Geometry check sheet. Reference: drawing and pictorial views, mm from the part's lowest x, y, z. Round coordinates to 2 decimals unless told otherwise and drop trailing zeros. Write each loop counter-clockwise with the first axis right and the second up, starting at its lowest first coordinate (ties: lowest second). Pieces come first, ordered by that corner, then holes.
Item 1: Section check A-A, the plane z = 39. Record the cut outline in (x, y) (3 decimals).
Item 2: Section check C-C, the plane z = 56. Record the cut outline in (x, y) (3 decimals).
Item 3: Depth check by flat-ended pin: pin 1 (1.5 mm diameter, centred on y = 1, z = 25, fed in from -X); pin 2 (1.9 mm diameter, centred on y = 2, z = 52, fed in from -X); pin 3 (3 mm diameter, centred on y = 2, z = 53, fed in from +X). Enter the tip coordinate at first touch or a pass-through.
Item 4: Section check B-B, the plane y = 4.5. Record the cut outline in (x, z) (3 decimals), plus the area to 3 significant figures.
Item 5: Section check D-D, the plane x = 49. Record the cut outline in (y, z).
Item 6: Material ranges on line 1 along X through (y, z) = (1.5, 30) (3 decimals); line 2 along X through (y, z) = (5.5, 62) (3 decimals); line 3 along Z through (x, y) = (55, 2.25), recorded low to high.
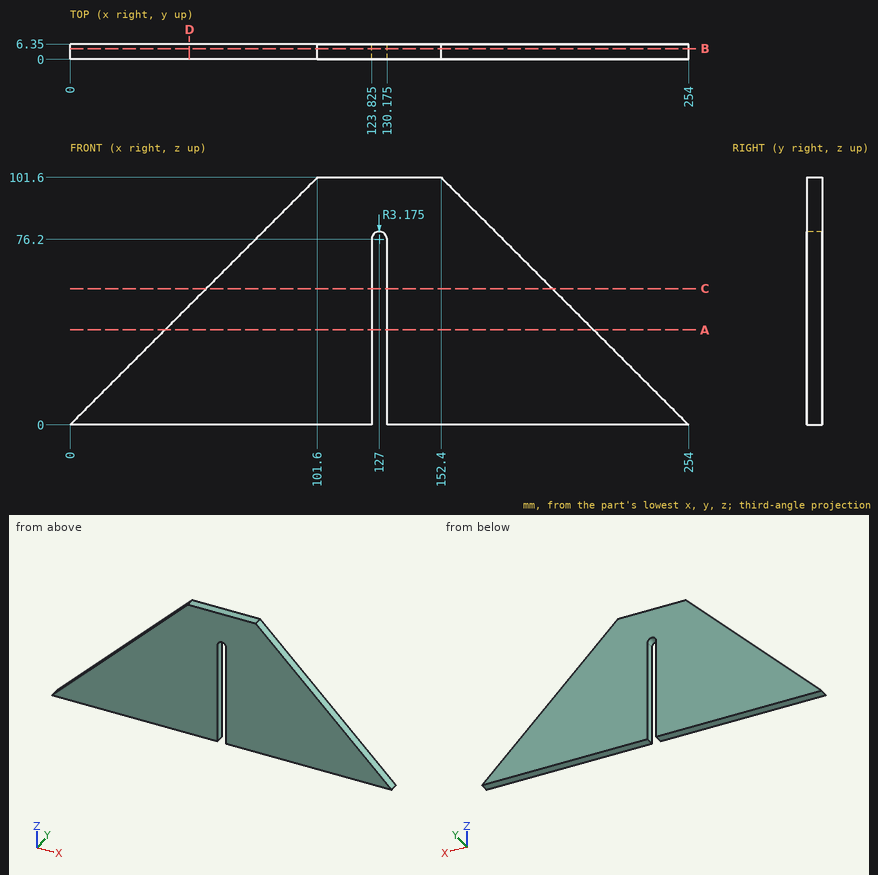
Values found:
1. outline: (39, 0) - (123.825, 0) - (123.825, 6.35) - (39, 6.35) - close; (130.175, 0) - (215, 0) - (215, 6.35) - (130.175, 6.35) - close
2. outline: (56, 0) - (123.825, 0) - (123.825, 6.35) - (56, 6.35) - close; (130.175, 0) - (198, 0) - (198, 6.35) - (130.175, 6.35) - close
3. pin 1: stops at x = 24.25
3. pin 2: stops at x = 51.05
3. pin 3: stops at x = 202.5
4. outline: (0, 0) - (123.825, 0) - (123.825, 76.2) arc R3.175 cw to (130.175, 76.2) - (130.175, 0) - (254, 0) - (152.4, 101.6) - (101.6, 101.6) - close
4. area: 15,000 mm2
5. outline: (0, 0) - (6.35, 0) - (6.35, 49) - (0, 49) - close
6. line 1: x = 30 to 123.825, 130.175 to 224
6. line 2: x = 62 to 123.825, 130.175 to 192
6. line 3: z = 0 to 55
